```python
from build123d import *

# Parameters (mm, degrees)
F0_R          = 8
F1_DEPTH      = 8
F1_DEPTH_BACK = 8
F3_D          = 5


with BuildPart() as f1:
    # F0 (on Front) → F1 (new body, two sides)
    with BuildSketch(Plane.XZ) as f1_sk:
        Polygon((-24, 0), (0, 0), (24, 0), (24, 8), (12.5, 8), (12.5, 44), (0, 44), (-12.5, 44), (-12.5, 8), (-24, 8), align=None)
        with Locations((0, 27)):
            Circle(F0_R, mode=Mode.SUBTRACT)
    extrude(amount=-F1_DEPTH)
    extrude(f1_sk.sketch, amount=F1_DEPTH_BACK)

    # F3 (through all)
    with Locations(Plane.XY.offset(8)):
        with Locations((-17.2336879396, 0), (17.2336879396, 0)):
            Hole(F3_D / 2)


solid = f1.part
```
Here's how the part is built. I have some questions about the finished solid (model axes, mm). A direction names the side the tool comes from. Coordinates: 2 decimals unless noted, no trailing zeros. Order: outer loops, then holes, each group sorted by start corner. A loop starts at its lowest first (then second) coordinate and runs counter-clockwise, first axis right, second up.
1) I need wall thicknesses on line 1 (Z direction, x = 0, y = 5); line 2 (X direction, y = 2, z = 8.5); line 3 (Z direction, x = -2, y = -3.5). Which ranges of each line are inside material? Lowest first, please.
2) We'd pull the mould along Y, two halves only. Please class faces 1 (the face through (0, 8, 17)), 2 (the face through (0, 0, 0)), 3 (the face through (0, -8, 17)), 4 (the face through (14.85, 0.75, 3.94)): +Y half, -Y half, draft (parallel to the pull), parting line (faces both ways), or undercut.
3) Which directions (+Z, -Z, +X, -X, +Y, -Y) give clear straight access to the entire face, cutting with the end or side of a thin tool? Please do faces 5 (the face through (0, 0, 44)), 6 (the face through (20, 2, 8)), 7 (the face through (-19, 2, 8)).
4) Imagine slicing it at A-A on y = 0. List the corners of the cut face in (x, z) for me, and give its area (3 significant figures).
5) Imagine slicing it at D-D on y = 4.5. List the corners of the cut face in (x, z) for me, and give its area (3 significant figures).
6) Will these pins go through, and if not, where does the flat tip stop? pin 1 (2 mm diameter, centred on y = 2, z = 31, fed in from -X); pin 2 (4 mm diameter, centred on y = -3, z = 39, fed in from +X); pin 3 (3.5 mm diameter, centred on x = 18, y = -4, fed in from +Z).
7) Imagine slicing it at B-B on x = 0. List the corners of the cut face in (y, z) for me.
8) Imagine slicing it at C-C on z = 27. List the corners of the cut face in (x, y) for me, and give its area (3 significant figures).
Response values:
1. line 1: z = 0 to 19, 35 to 44
1. line 2: x = -12.5 to 12.5
1. line 3: z = 0 to 19.25, 34.75 to 44
2. face 1: +Y half
2. face 2: draft
2. face 3: -Y half
2. face 4: undercut
3. face 5: +Z, +X, -X, +Y, -Y
3. face 6: +Z, +X, +Y, -Y
3. face 7: +Z, -X, +Y, -Y
4. outline: (-24, 0) - (-19.73, 0) - (-19.73, 8) - (-24, 8) - close; (-14.73, 0) - (14.73, 0) - (14.73, 8) - (12.5, 8) - (12.5, 44) - (-12.5, 44) - (-12.5, 8) - (-14.73, 8) - close; (19.73, 0) - (24, 0) - (24, 8) - (19.73, 8) - close; hole circle Ø16 at (0, 27)
4. area: 1,000 mm2
5. outline: (-24, 0) - (24, 0) - (24, 8) - (12.5, 8) - (12.5, 44) - (-12.5, 44) - (-12.5, 8) - (-24, 8) - close; hole circle Ø16 at (0, 27)
5. area: 1,080 mm2
6. pin 1: stops at x = -12.5
6. pin 2: stops at x = 12.5
6. pin 3: stops at z = 8
7. outline: (-8, 0) - (8, 0) - (8, 19) - (-8, 19) - close; (-8, 35) - (8, 35) - (8, 44) - (-8, 44) - close
8. outline: (-12.5, -8) - (-8, -8) - (-8, 8) - (-12.5, 8) - close; (8, -8) - (12.5, -8) - (12.5, 8) - (8, 8) - close
8. area: 144 mm2
